Part model, mm, in its own coordinate system. Face numbers are marked on the shaded views. A direction names the side the tool comes from. Coordinates: 2 decimals unless noted, no trailing zeros. Order: outer loops, then holes, each group sorted by start corner. A loop starts at its lowest first (then second) coordinate and runs counter-clockwise, first axis right, second up. Notation, with made-up numbers: (79.25, 77) - (112.25, 77) arc R14 cw to (112.25, 93) - close; hole circle Ø10 at (12.25, 38). An arc over 180 degrees is marked (long way). Use a Markdown table: item, result. Add a question column.
1) Saw through at D-D on z = 2.5. List the corners of the cut face in (x, y).
2) Tool access for the marked faces 4, 5, 6 and 7: list every direction of +Z, -Z, +X, -X, +Y, -Y with a clear straight run to the whole face (end or side of a thin tool).
3) Saw through at A-A on z = 7. List the corners of the cut face in (x, y).
4) Two-plate mould, pull along Z, no slides. Class the marked faces 1, 2 and 3: +Z half, -Z half, draft (parallel to the pull), parting line (faces both ways), or undercut.
5) Wall check: L1, parallel to X at y = 13.25, z = 2; L2, parallel to X at y = 6.5, z = 10.5; L3, parallel to Z at x = 15.24, y = 5.5. Give the ranges that are in metal, low to high. Write a range as [from, to].
6) Saw through at B-B on x = -3.5. List the corners of the cut face in (y, z), then the cut area to 3 significant figures.
7) Drop flat-ended pins along their axis: P1, Ø1.9, axis at y = 10, z = 16, coming from the +X side; P2, Ø6, axis at y = 8.5, z = 6.5, coming from the +X side; P3, Ø11.5, axis at x = 16.5, z = 19, coming from the +Y side; P4, Ø3.5, axis at y = 10.67, z = 4.19, coming from the +X side. Give the stop position or say it passes through.
8) Saw through at C-C on y = 4.75. List the corners of the cut face in (x, z), then the cut area to 3 significant figures.
```python
from build123d import *

# Parameters (mm, degrees)
BOSS_EXTRUDE1_DEPTH = 25.4
SKETCH6_R           = 4.25
CUT_EXTRUDE1_DEPTH  = 14.97
SKETCH12_R          = 2.5527
CUT_EXTRUDE2_DEPTH  = 8.62
CUT_EXTRUDE3_DEPTH  = 14.97
SKETCH16_R          = 2.249932
CUT_EXTRUDE8_DEPTH  = 30.62966793


with BuildPart() as part:
    # Sketch1 → Boss-Extrude1 (new body)
    with BuildSketch(Plane.XY):
        Polygon((-20.052587871, 0), (-20.052587871, 7.62), (-9.577080059, 7.62), (-9.577080059, 13.97), (9.577080059, 13.97), (9.577080059, 7.62), (20.052587871, 7.62), (20.052587871, 0), align=None)
    extrude(amount=BOSS_EXTRUDE1_DEPTH)

    # Sketch6 → Cut-Extrude1 (cut, through all)
    with BuildSketch(Plane(origin=(0, 13.97, 0), x_dir=(1, 0, 0), z_dir=(0, 1, 0))):
        with Locations((0, -15.788153465)):
            Circle(SKETCH6_R)
    extrude(amount=-CUT_EXTRUDE1_DEPTH, mode=Mode.SUBTRACT)

    # Sketch12 → Cut-Extrude2 (cut, through all)
    with BuildSketch(Plane(origin=(0, 7.62, 0), x_dir=(1, 0, 0), z_dir=(0, 1, 0))):
        with Locations((-15.141300214, -16.51)):
            Circle(SKETCH12_R)
        with Locations((15.24, -16.556540888)):
            Circle(SKETCH12_R)
    extrude(amount=-CUT_EXTRUDE2_DEPTH, mode=Mode.SUBTRACT)

    # Sketch14 → Cut-Extrude3 (cut, through all)
    with BuildSketch(Plane(origin=(0, 13.97, 0), x_dir=(1, 0, 0), z_dir=(0, 1, 0))):
        Polygon((-1.27, 0), (1.27, 0), (1.27, -11.699930965), (0, -11.538153465), (-1.27, -11.699930965), align=None)
    extrude(amount=-CUT_EXTRUDE3_DEPTH, mode=Mode.SUBTRACT)

    # Sketch16 → Cut-Extrude8 (cut, through all)
    with BuildSketch(Plane(origin=(9.577080059, 0, 0), x_dir=(0, 0, -1), z_dir=(1, 0, 0))):
        with Locations((-4.189047087, 10.668)):
            Circle(SKETCH16_R)
    extrude(amount=-CUT_EXTRUDE8_DEPTH, mode=Mode.SUBTRACT)


solid = part.part
```
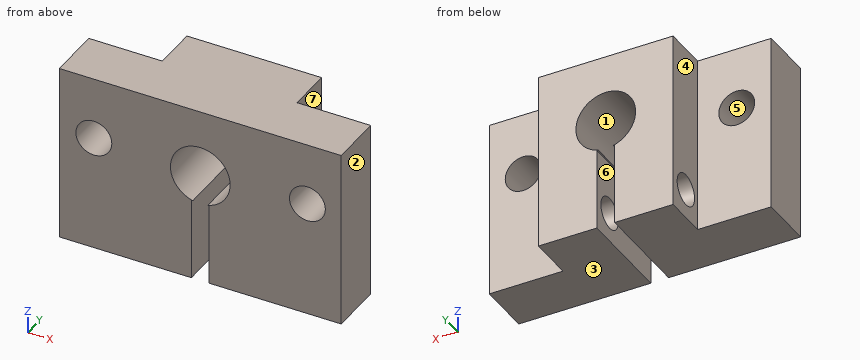
Results are:
| question | item | result |
|---|---|---|
| 1 | outline | (-20.05, 0) - (-1.27, 0) - (-1.27, 9.18) - (-9.58, 9.18) - (-9.58, 7.62) - (-20.05, 7.62) - close; (-9.58, 12.15) - (-1.27, 12.15) - (-1.27, 13.97) - (-9.58, 13.97) - close; (1.27, 0) - (20.05, 0) - (20.05, 7.62) - (9.58, 7.62) - (9.58, 9.18) - (1.27, 9.18) - close; (1.27, 12.15) - (9.58, 12.15) - (9.58, 13.97) - (1.27, 13.97) - close |
| 2 | face 4 | +Z, -Z, -X, +Y |
| 2 | face 5 | +Y, -Y |
| 2 | face 6 | -Z, +Y, -Y |
| 2 | face 7 | +Z, -Z, +X, +Y |
| 3 | outline | (-20.05, 0) - (-1.27, 0) - (-1.27, 13.97) - (-9.58, 13.97) - (-9.58, 7.62) - (-20.05, 7.62) - close; (1.27, 0) - (20.05, 0) - (20.05, 7.62) - (9.58, 7.62) - (9.58, 13.97) - (1.27, 13.97) - close |
| 4 | face 1 | undercut |
| 4 | face 2 | draft |
| 4 | face 3 | -Z half |
| 5 | L1 | [-9.58, -1.27], [1.27, 9.58] |
| 5 | L2 | [-20.05, -1.27], [1.27, 20.05] |
| 5 | L3 | [0, 14], [19.11, 25.4] |
| 6 | outline | (0, 0) - (13.97, 0) - (13.97, 13.38) - (0, 13.38) - close; (0, 18.2) - (13.97, 18.2) - (13.97, 25.4) - (0, 25.4) - close; hole circle Ø4.5 at (10.67, 4.19) |
| 6 | area | 272 mm2 |
| 7 | P1 | x = 9.58 |
| 7 | P2 | x = 20.05 |
| 7 | P3 | y = 7.62 |
| 7 | P4 | through |
| 8 | outline | (-20.05, 0) - (-1.27, 0) - (-1.27, 11.7) - (-1.07, 11.67) arc R4.25 cw (long way) to (1.07, 11.67) - (1.27, 11.7) - (1.27, 0) - (20.05, 0) - (20.05, 25.4) - (-20.05, 25.4) - close; hole circle Ø5.11 at (-15.14, 16.51); hole circle Ø5.11 at (15.24, 16.56) |
| 8 | area | 892 mm2 |
